Here's how the part is built. I have some questions about the finished solid (model axes, mm). Face numbers are marked on the shaded views. A direction names the side the tool comes from. Coordinates: 2 decimals unless noted, no trailing zeros. Loops run counter-clockwise (first coordinate to the right, second up) from the corner with the lowest first, then second, coordinate; pieces in that order, holes last. Notation, with made-up numbers: (67.5, 62.25) - (112.5, 62.25) arc R22 ccw to (112.5, 78.25) - close; hole circle Ø8 at (-15, 64.25). An arc over 180 degrees is marked (long way). Use a Markdown table: item, result.
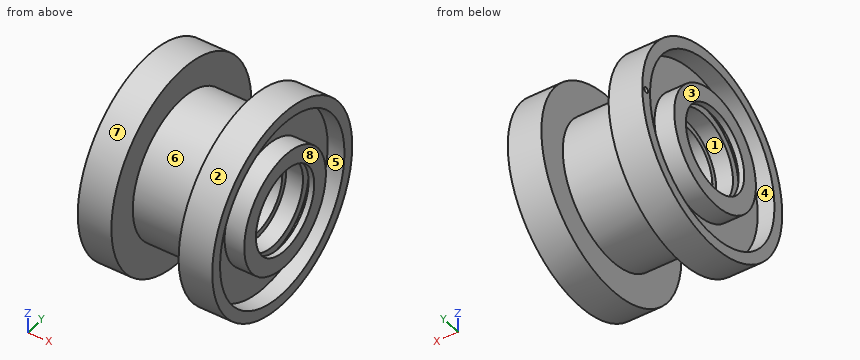
```python
from build123d import *

# Parameters (mm, degrees)
SZKIC2_R                   = 0.5
WYTNIJ_WYCI_GNI_CIE1_DEPTH = 1


with BuildPart() as part:
    # Szkic1 → Obrót1 (revolve)
    with BuildSketch(Plane.XY, mode=Mode.PRIVATE) as obr_t1_sk:
        Polygon((-6, 12.5), (6, 12.5), (6, 18), (12, 18), (12, 16), (9, 16), (9, 10.5), (12.5, 10.5), (12.5, 7.5), (11.5, 7.5), (11.5, 8.9), (10.5, 8.9), (10.5, 7.5), (7.5, 7.5), (7.5, 6.5), (-7.5, 6.5), (-7.5, 7.5), (-10.5, 7.5), (-10.5, 8.9), (-11.5, 8.9), (-11.5, 7.5), (-12.5, 7.5), (-12.5, 10.5), (-9, 10.5), (-9, 16), (-12, 16), (-12, 18), (-6, 18), align=None)
    revolve(obr_t1_sk.sketch.rotate(Axis((-12.5, 0, 0), (1, 0, 0)), 90), axis=Axis((-12.5, 0, 0), (1, 0, 0)))

    # Szkic2 → Wytnij-wyciągnięcie1 (cut)
    with BuildSketch(Plane.ZY.offset(12)):
        with Locations((0, 17)):
            Circle(SZKIC2_R)
    extrude(amount=-WYTNIJ_WYCI_GNI_CIE1_DEPTH, mode=Mode.SUBTRACT)


solid = part.part
```
Q1. I want a section at C-C, the plane x = -8.5. Write out the boundary of the cut face in (y, z).
Check values:
| item | result |
|---|---|
| outline | circle Ø36 at (0, 0); hole circle Ø15 at (0, 0) |
Q2. Please list where these lines run through material, in increasing order: L1, parallel to Y at x = -10.75, z = 0; L2, parallel to Y at x = -11.15, z = 0; L3, parallel to Y at x = 11.8, z = 0. Write a range as from..to.
Check values:
| item | result |
|---|---|
| L1 | -18..-16, -10.5..-8.9, 8.9..10.5, 16..18 |
| L2 | -18..-16, -10.5..-8.9, 8.9..10.5, 16..16.5, 17.5..18 |
| L3 | -18..-16, -10.5..-7.5, 7.5..10.5, 16..18 |
Q3. I want a section at A-A, the plane z = 14.5. Write out the boundary of the cut face in (x, y).
Check values:
| item | result |
|---|---|
| outline | (-12, -10.67) - (-6, -10.67) - (-6, 10.67) - (-12, 10.67) - (-12, 6.76) - (-9, 6.76) - (-9, -6.76) - (-12, -6.76) - close; (6, -10.67) - (12, -10.67) - (12, -6.76) - (9, -6.76) - (9, 6.76) - (12, 6.76) - (12, 10.67) - (6, 10.67) - close |
Q4. I want a section at B-B, the plane y = 15.5. Write out the boundary of the cut face in (x, z), then the cut area to 3 significant figures.
Check values:
| item | result |
|---|---|
| outline | (-12, -9.15) - (-6, -9.15) - (-6, 9.15) - (-12, 9.15) - (-12, 3.97) - (-9, 3.97) - (-9, -3.97) - (-12, -3.97) - close; (6, -9.15) - (12, -9.15) - (12, -3.97) - (9, -3.97) - (9, 3.97) - (12, 3.97) - (12, 9.15) - (6, 9.15) - close |
| area | 172 mm^2 |
Q5. If we mould it in two halves opening along Z, with no side actions, what happens to the marked faces 1, 2 and 3? For each: pulls with the +Z half, pulls with the -Z half, needs draft (parallel to the pull), parting line crosses it, or undercut.
Check values:
| item | result |
|---|---|
| face 1 | undercut |
| face 2 | parting line crosses it |
| face 3 | needs draft |
Q6. Which directions (+Z, -Z, +X, -X, +Y, -Y) give clear straight access to the entire face, cutting with the end or side of a thin tool? Please do the marked faces 4, 5, 6, 7 and 8.
Check values:
| item | result |
|---|---|
| face 4 | -X |
| face 5 | +X |
| face 6 | none |
| face 7 | +X, -X |
| face 8 | +Z, -Z, +X, +Y, -Y |
Q7. I want a section at D-D, the plane y = 10. Write out the boundary of the cut face in (x, z).
Check values:
| item | result |
|---|---|
| outline | (-12.5, -3.2) - (-9, -3.2) - (-9, -12.49) - (-12, -12.49) - (-12, -14.97) - (-6, -14.97) - (-6, -7.5) - (6, -7.5) - (6, -14.97) - (12, -14.97) - (12, -12.49) - (9, -12.49) - (9, -3.2) - (12.5, -3.2) - (12.5, 3.2) - (9, 3.2) - (9, 12.49) - (12, 12.49) - (12, 14.97) - (6, 14.97) - (6, 7.5) - (-6, 7.5) - (-6, 14.97) - (-12, 14.97) - (-12, 12.49) - (-9, 12.49) - (-9, 3.2) - (-12.5, 3.2) - close |
Q8. Will these pins go through, and if not, where does the flat tip stop? P1, Ø1.1, axis at y = 17, z = 0, coming from the -X side; P2, Ø5, axis at x = -2.5, y = 5.5, coming from the +Z side; P3, Ø8, axis at y = 9.5, z = 9, coming from the +X side; P4, Ø6, axis at x = 7, y = 12, coming from the -Z side.
Check values:
| item | result |
|---|---|
| P1 | x = -12 |
| P2 | z = 12.13 |
| P3 | x = 12.5 |
| P4 | z = -15.59 |
